For this review, take the finished solid that the model builds, in its own axes (mm). A direction names the side the tool comes from. Coordinates: 2 decimals unless noted, no trailing zeros. Loops run counter-clockwise (first coordinate to the right, second up) from the corner with the lowest first, then second, coordinate; pieces in that order, holes last. Notation, with made-up numbers: M 78.25,-10 L 90.25,-10 A15 ccw 90.25,5 Z; hole C 35.5,65 d5. An arc over 180 degrees is marked long. Answer as a JSON object with one key per item and string values. Group by question number.
Item 1: Add section A-A (y = 25.5). State the section outline as (x, z) points, then the cut area to 3 significant figures.
Item 2: Add section D-D (z = 3). Count the separate pieces of the cut face and the enclosed holes in it, then the cut area to 3 significant figures.
Item 3: Tool access review of faces 3 (the face through (-61.15, 20, 6)), 4 (the face through (25, 20.5, 2)), 5 (the face through (-60, 18.496, 5)): name each direction out of +Z, -Z, +X, -X, +Y, -Y from which nothing blocks a thin tool from reaching the whole face with its end or side.
Item 4: Wall thickness on L1, parallel to X at y = 6.5, z = 2.25; L2, parallel to Y at x = -3, z = 1; L3, parallel to X at y = 21, z = 7.75: over which ranges is each line inside the solid? List them lowest first. Write a range as from..to.
Item 5: Insertion check: pin 1 (4 mm diameter, centred on x = 16.5, z = 6.5, fed in from +Y); pin 2 (1 mm diameter, centred on x = -13.5, z = 6, fed in from -Y); pin 3 (1.5 mm diameter, centred on x = 25.5, z = 7, fed in from +Y); pin 4 (1 mm diameter, centred on x = 18.5, y = 5, fed in from -Z). Each pin has a flat end and moves straight along its axis. Give the tip position at first contact, or say it passes through.
Item 6: Mouldability with a two-part tool opening along X and no side actions: class faces 1 (the face through (-59.15, 20, 6)), 2 (the face through (-64, 18.496, 5)) as +X half, -X half, draft (parallel to the pull), parting line (faces both ways), or undercut.
from build123d import *

# Parameters (mm, degrees)
BOSS_EXTRUDE2_DEPTH  = 11
BOSS_EXTRUDE3_DEPTH  = 5
SKETCH2_W            = 30.2
SKETCH2_H            = 1
BOSS_EXTRUDE4_DEPTH  = 25.5
SKETCH1_W            = 7.8
SKETCH1_H            = 14.5
BOSS_EXTRUDE5_DEPTH  = 11
SKETCH3_W            = 11.2
SKETCH3_H            = 11
BOSS_EXTRUDE6_DEPTH  = 5
SKETCH4_W            = 31.1
SKETCH4_H            = 4
CUT_EXTRUDE1_DEPTH   = 10
SKETCH5_W            = 32
SKETCH5_H            = 5
BOSS_EXTRUDE7_DEPTH  = 1
BOSS_EXTRUDE8_DEPTH  = 62.24
SKETCH8_W            = 0.9
SKETCH8_H            = 1
BOSS_EXTRUDE9_DEPTH  = 6
SKETCH9_W            = 0.9
SKETCH9_H            = 10.000488142
BOSS_EXTRUDE10_DEPTH = 62.26
SKETCH10_W           = 52.24
SKETCH10_H           = 1
BOSS_EXTRUDE11_DEPTH = 6
SKETCH11_R           = 81.7
SKETCH11_R_2         = 70.15
CUT_EXTRUDE2_DEPTH   = 6.2
SKETCH12_W           = 11
SKETCH12_H           = 1
SKETCH12_W_2         = 0.9
SKETCH12_H_2         = 10
BOSS_EXTRUDE12_DEPTH = 2.91
SKETCH14_W           = 2
SKETCH14_H           = 11
BOSS_EXTRUDE13_DEPTH = 2
SKETCH15_W           = 2
SKETCH15_H           = 11
BOSS_EXTRUDE14_DEPTH = 2
SKETCH20_RX          = 7.25
SKETCH20_RY          = 5
CUT_EXTRUDE3_DEPTH   = 10
SKETCH21_W           = 6
SKETCH21_H           = 8
CUT_EXTRUDE4_DEPTH   = 1
SKETCH22_W           = 4
SKETCH22_H           = 8
CUT_EXTRUDE5_DEPTH   = 1


with BuildPart() as part:
    # Sketch1_3 → Boss-Extrude2 (new body)
    with BuildSketch(Plane.XY):
        Polygon((0, 31.5), (0, 0), (32, 0), (32, 31.5), (31.1, 31.5), (31.1, 6), (0.9, 6), (0.9, 31.5), align=None)
    extrude(amount=BOSS_EXTRUDE2_DEPTH)

    # Sketch1_4 → Boss-Extrude3 (add)
    with BuildSketch(Plane.XY):
        Polygon((0.9, 31.5), (0.9, 20.5), (12.1, 20.5), (19.9, 20.5), (31.1, 20.5), (31.1, 31.5), align=None)
    extrude(amount=BOSS_EXTRUDE3_DEPTH)

    # Sketch2 → Boss-Extrude4 (add)
    with BuildSketch(Plane(origin=(0, 6, 0), x_dir=(1, 0, 0), z_dir=(0, 1, 0))):
        with Locations((16, -10.5)):
            Rectangle(SKETCH2_W, SKETCH2_H)
    extrude(amount=BOSS_EXTRUDE4_DEPTH)

    # Sketch1 → Boss-Extrude5 (add)
    with BuildSketch(Plane.XY):
        with Locations((16, 13.25)):
            Rectangle(SKETCH1_W, SKETCH1_H)
    extrude(amount=BOSS_EXTRUDE5_DEPTH)

    # Sketch3 → Boss-Extrude6 (add)
    with BuildSketch(Plane(origin=(0, 0, 10), x_dir=(-1, 0, 0), z_dir=(0, 0, -1))):
        with Locations((-6.5, 11.5)):
            Rectangle(SKETCH3_W, SKETCH3_H)
        with Locations((-25.5, 11.5)):
            Rectangle(SKETCH3_W, SKETCH3_H)
    extrude(amount=BOSS_EXTRUDE6_DEPTH)

    # Sketch4 → Cut-Extrude1 (cut)
    with BuildSketch(Plane(origin=(0, 31.5, 0), x_dir=(1, 0, 0), z_dir=(0, 1, 0))):
        with Locations((15.55, -2.4)):
            Rectangle(SKETCH4_W, SKETCH4_H)
    extrude(amount=-CUT_EXTRUDE1_DEPTH, mode=Mode.SUBTRACT)

    # Sketch5 → Boss-Extrude7 (add)
    with BuildSketch(Plane(origin=(0, 31.5, 0), x_dir=(1, 0, 0), z_dir=(0, 1, 0))):
        with Locations((16, -2.5)):
            Rectangle(SKETCH5_W, SKETCH5_H)
    extrude(amount=BOSS_EXTRUDE7_DEPTH)

    # Sketch7 → Boss-Extrude8 (add)
    with BuildSketch(Plane.ZY):
        Polygon((5, 20.496183522), (5, 21.5), (4.4, 21.5), (0.4, 21.5), (0, 21.5), (0, 20.496183522), align=None)
        Polygon((5, 31.5), (5, 32.5), (0, 32.5), (0, 31.5), (0.4, 31.5), (4.4, 31.5), align=None)
    extrude(amount=BOSS_EXTRUDE8_DEPTH)

    # Sketch8 → Boss-Extrude9 (add)
    with BuildSketch(Plane.XY.offset(5)):
        with Locations((0.45, 32)):
            Rectangle(SKETCH8_W, SKETCH8_H)
    extrude(amount=BOSS_EXTRUDE9_DEPTH)

    # Sketch9 → Boss-Extrude10 (add)
    with BuildSketch(Plane.ZY):
        Polygon((11, 20.496183522), (11, 21.499511858), (10.1, 21.499511858), (5, 21.499511858), (5, 20.496183522), align=None)
        with Locations((10.55, 26.499755929)):
            Rectangle(SKETCH9_W, SKETCH9_H)
    extrude(amount=BOSS_EXTRUDE10_DEPTH)

    # Sketch10 → Boss-Extrude11 (add)
    with BuildSketch(Plane.XY.offset(5)):
        with Locations((-36.12, 32)):
            Rectangle(SKETCH10_W, SKETCH10_H)
    extrude(amount=BOSS_EXTRUDE11_DEPTH)

    # Sketch11 → Cut-Extrude2 (cut)
    with BuildSketch(Plane(origin=(0, 0, 0), x_dir=(-1, 0, 0), z_dir=(0, 0, -1))):
        with Locations((71.241875, 77.677250508)):
            Circle(SKETCH11_R)
        with Locations((71.241875, 77.677250508)):
            Circle(SKETCH11_R_2, mode=Mode.SUBTRACT)
    extrude(amount=-CUT_EXTRUDE2_DEPTH, mode=Mode.SUBTRACT)

    # Sketch12 → Boss-Extrude12 (add)
    with BuildSketch(Plane.ZY.offset(62.24)):
        with Locations((5.5, 32)):
            Rectangle(SKETCH12_W, SKETCH12_H)
        with Locations((10.55, 26.5)):
            Rectangle(SKETCH12_W_2, SKETCH12_H_2)
        Polygon((11, 20.496183522), (11, 21.5), (10.1, 21.5), (5, 21.5), (5, 21.499511858), (5, 20.496183522), align=None)
        Polygon((5, 21.499511858), (5, 21.5), (0, 21.5), (0, 20.496183522), (5, 20.496183522), align=None)
    extrude(amount=BOSS_EXTRUDE12_DEPTH)

    # Sketch14 → Boss-Extrude13 (add)
    with BuildSketch(Plane(origin=(0, 20.496183522, 0), x_dir=(-1, 0, 0), z_dir=(0, -1, 0))):
        with Locations((64.15, -5.5)):
            Rectangle(SKETCH14_W, SKETCH14_H)
        with Locations((60.15, -5.5)):
            Rectangle(SKETCH14_W, SKETCH14_H)
    extrude(amount=BOSS_EXTRUDE13_DEPTH)

    # Sketch15 → Boss-Extrude14 (add)
    with BuildSketch(Plane(origin=(0, 32.5, 0), x_dir=(1, 0, 0), z_dir=(0, 1, 0))):
        with Locations((-64.15, -5.5)):
            Rectangle(SKETCH15_W, SKETCH15_H)
        with Locations((-60.15, -5.5)):
            Rectangle(SKETCH15_W, SKETCH15_H)
    extrude(amount=BOSS_EXTRUDE14_DEPTH)

    # Sketch20 → Cut-Extrude3 (cut)
    with BuildSketch(Plane(origin=(19.9, 0, 0), x_dir=(0, 0, -1), z_dir=(1, 0, 0))):
        with Locations(Location((0, 13.25), (0, 0, -90))):
            Ellipse(SKETCH20_RX, SKETCH20_RY)
    extrude(amount=-CUT_EXTRUDE3_DEPTH, mode=Mode.SUBTRACT)

    # Sketch21 → Cut-Extrude4 (cut)
    with BuildSketch(Plane.XY.offset(11)):
        with Locations((5.9, 27.5)):
            Rectangle(SKETCH21_W, SKETCH21_H)
        with Locations((27, 27.5)):
            Rectangle(SKETCH21_W, SKETCH21_H)
    extrude(amount=-CUT_EXTRUDE4_DEPTH, mode=Mode.SUBTRACT)

    # Sketch22 → Cut-Extrude5 (cut)
    with BuildSketch(Plane(origin=(32, 0, 0), x_dir=(0, 0, -1), z_dir=(1, 0, 0))):
        with Locations((-2.4, 26.5)):
            Rectangle(SKETCH22_W, SKETCH22_H)
    extrude(amount=-CUT_EXTRUDE5_DEPTH, mode=Mode.SUBTRACT)


solid = part.part
From the geometry:
{
 "1": {"outline": "M -65.15,10.1 L 0,10.1 L 0,4.4 L 32,4.4 L 32,11 L 30,11 L 30,10 L 31.1,10 L 31.1,5 L 0.9,5 L 0.9,10 L 2.9,10 L 2.9,11 L -65.15,11 Z; M 0,0 L 32,0 L 32,0.4 L 0,0.4 Z; M 8.9,10 L 24,10 L 24,11 L 8.9,11 Z", "area": "120 mm²"},
 "2": {"separate pieces": "4", "enclosed holes": "1", "area": "421 mm²"},
 "3": {"face 3": "+Z, -Z, -Y", "face 4": "-Z", "face 5": "+Z, -Z, -X, -Y"},
 "4": {"L1": "x = 0..0.9, 12.1..19.9, 31.1..32", "L2": "y = 20.5..21.5, 31.5..32.5", "L3": "x = -65.15..0.9, 31.1..32"},
 "5": {"pin 1": "stops at y = 32.5", "pin 2": "stops at y = 20.5", "pin 3": "stops at y = 17", "pin 4": "stops at z = 0"},
 "6": {"face 1": "undercut", "face 2": "draft"}
}
